Geometry: final body of the model. Coordinates: model frame, mm. A direction names the side the tool comes from. Coordinates: 2 decimals unless noted, no trailing zeros. Loops run counter-clockwise (first coordinate to the right, second up) from the corner with the lowest first, then second, coordinate; pieces in that order, holes last. Notation, with made-up numbers: (14.5, -11.5) -> (44.5, -11.5) arc R27 cw to (44.5, 17.5) -> close; hole circle Ø3 at (-15.5, -30.5). An arc over 180 degrees is marked (long way). One line per item, written item: value. Start each with the question number.
Item 1: Section query D-D on z = 3. Return loops of the section in (x, y), then the cut area to 3 significant figures.
Item 2: Section query C-C on y = 14.95. Give the number of separate pieces and of enclosed holes in the cut face, then the cut area to 3 significant figures.
Item 3: Ray query, probe 1 along Y at (x, z) = (3.2, 0.4); probe 2 along Z at (x, y) = (4.25, 9.5); probe 3 along Y at (x, z) = (3.2, 3.6). Return the intervals inside material, ascending. Write a range as from..to.
Item 4: Set-up query: faces 4 (the flat face through (2, 2, 3.35)), 5 (the flat face through (10.7, 14.8, 0.5)), 6 (the cylindrical face through (11.79, 11.76, 0.49)), 7 (the flat face through (13.353, 9, -2)). Return all of +Z, -Z, +X, -X, +Y, -Y with unobstructed straight access to the full face (end or side cutting, diameter ignored); none if empty.
Item 5: Section query A-A on x = 10.2. Return loops of the section in (y, z).
Item 6: Contact query for flat-ended pins moving along their axis: pin 1 Ø0.6 at (y, z) = (15, 1) entering from -X; pin 2 Ø1.6 at (y, z) = (11.5, -1.5) entering from -X; pin 3 Ø1.2 at (x, y) = (2, 2.5) entering from -Z; pin 4 Ø2 at (x, y) = (3.2, 2.95) entering from +Z. Output: stop coordinate, or through.
Item 7: Mould query, pull axis Y, two halves, no side actions, for faces 1 (the cylindrical face through (4.265, 2.396, 3.646)), 2 (the flat face through (14.24, 8.726, 2.806)), 3 (the flat face through (11.4, 17.1, 0.5)). Classes: +Y half, -Y half, draft (parallel to the pull), parting line (faces both ways), or undercut.
from build123d import *

# Parameters (mm, degrees)
BOSS_EXTRUDE1_DEPTH                             = 15.4
CUT_EXTRUDE2_REACH                              = 25.978
SKETCH3_W                                       = 7.5
SKETCH3_H                                       = 11.5
BOSS_EXTRUDE3_REACH                             = 25.978
SKETCH4_W                                       = 0.8
SKETCH4_H                                       = 6.2
SKETCH4_W_2                                     = 2.8
SKETCH4_H_2                                     = 17.7
SKETCH10_W                                      = 4
SKETCH10_H                                      = 1
CUT_EXTRUDE4_DEPTH                              = 16.3
BOSS_EXTRUDE4_DEPTH                             = 0.8
CSK_FOR_M2_FLAT_HEAD_MACHINE_SCREW3_D           = 2.4
CSK_FOR_M2_FLAT_HEAD_MACHINE_SCREW3_CSINK_D     = 4.4
CSK_FOR_M2_FLAT_HEAD_MACHINE_SCREW3_CSINK_ANGLE = 90
MOVE_FACE1_BY                                   = 0.6
SKETCH3_2_W                                     = 7.5
SKETCH3_2_H                                     = 11.5
BOSS_EXTRUDE6_DEPTH                             = 0.8
CHAMFER1_SIZE                                   = 2.5
CHAMFER1_SIZE2                                  = 4
SKETCH12_W                                      = 2.0475
SKETCH12_H                                      = 3.18
BOSS_EXTRUDE5_DEPTH                             = 17.7
SKETCH11_R                                      = 1.75
CUT_EXTRUDE5_DEPTH                              = 25.580050854
BOSS_EXTRUDE7_DEPTH                             = 1
SKETCH16_W                                      = 8.2
SKETCH16_H                                      = 5.5
CUT_EXTRUDE6_DEPTH                              = 0.5
FILLET5_R                                       = 0.5
FILLET6_R                                       = 0.8


with BuildPart() as part:
    # Sketch2 → Boss-Extrude1 (new body)
    with BuildSketch(Plane(origin=(0, 0, 0), x_dir=(0, 0, -1), z_dir=(1, 0, 0))):
        Polygon((0, 0), (-4.95, 0), (-4.95, 17.7), (-4.15, 17.7), (-4.15, 0.8), (-1, 0.8), (-1, 17.7), (0, 17.7), align=None)
    extrude(amount=BOSS_EXTRUDE1_DEPTH)

    # Sketch3 → Cut-Extrude2 (cut, up to next)
    with BuildSketch(Plane.XY.offset(4.95), mode=Mode.PRIVATE) as cut_extrude2_sk1:
        with Locations((3.75, 11.95)):
            Rectangle(SKETCH3_W, SKETCH3_H)
    cut_extrude2_tool1 = extrude(cut_extrude2_sk1.sketch, amount=-CUT_EXTRUDE2_REACH, mode=Mode.PRIVATE) & part.part
    add(cut_extrude2_tool1.solids().sort_by_distance((3.75, 11.95, 4.95))[0], mode=Mode.SUBTRACT)

    # Sketch4 → Boss-Extrude3 (add, up to next)
    with BuildSketch(Plane.XY.offset(4.95), mode=Mode.PRIVATE) as boss_extrude3_sk1:
        with Locations((0.4, 3.1)):
            Rectangle(SKETCH4_W, SKETCH4_H)
    boss_extrude3_tool1 = extrude(boss_extrude3_sk1.sketch, amount=-BOSS_EXTRUDE3_REACH, mode=Mode.PRIVATE) - part.part
    # Sketch4 → Boss-Extrude3 (add, up to next)
    with BuildSketch(Plane.XY.offset(4.95), mode=Mode.PRIVATE) as boss_extrude3_sk2:
        with Locations((14, 8.85)):
            Rectangle(SKETCH4_W_2, SKETCH4_H_2)
    boss_extrude3_tool2 = extrude(boss_extrude3_sk2.sketch, amount=-BOSS_EXTRUDE3_REACH, mode=Mode.PRIVATE) - part.part
    add(boss_extrude3_tool1.solids().sort_by_distance((0.4, 3.1, 4.95))[0])
    add(boss_extrude3_tool2.solids().sort_by_distance((14, 8.85, 4.95))[0])

    # Sketch10 → Cut-Extrude4 (cut)
    with BuildSketch(Plane(origin=(0, 17.7, 0), x_dir=(1, 0, 0), z_dir=(0, 1, 0))):
        with Locations((10.2, -0.5)):
            Rectangle(SKETCH10_W, SKETCH10_H)
    extrude(amount=-CUT_EXTRUDE4_DEPTH, mode=Mode.SUBTRACT)

    # Sketch6 → Boss-Extrude4 (add)
    with BuildSketch(Plane(origin=(0, 0, 4.15), x_dir=(-1, 0, 0), z_dir=(0, 0, -1))):
        with BuildLine():
            Line((-0.8, 0.8), (-5.05, 0.8))
            Line((-5.05, 0.8), (-5.05, 2.95))
            ThreePointArc((-5.05, 2.95), (-4.508147545, 4.258147545), (-3.2, 4.8))
            Line((-3.2, 4.8), (-0.8, 4.8))
            Line((-0.8, 4.8), (-0.8, 0.8))
        make_face()
    extrude(amount=BOSS_EXTRUDE4_DEPTH)

    # CSK for M2 Flat Head Machine Screw3 (through all)
    with Locations(Plane(origin=(10.2, 14.95, 4.95), x_dir=(0, 1, 0), z_dir=(0, 0, 1))):
        with Locations((0, 0), (-12, 7)):
            CounterSinkHole(CSK_FOR_M2_FLAT_HEAD_MACHINE_SCREW3_D / 2, CSK_FOR_M2_FLAT_HEAD_MACHINE_SCREW3_CSINK_D / 2, counter_sink_angle=CSK_FOR_M2_FLAT_HEAD_MACHINE_SCREW3_CSINK_ANGLE)

    # Move Face1: a face moved inward by 0.6
    extrude(part.faces().sort_by_distance((4.1, 17.7, 0.5))[0], amount=MOVE_FACE1_BY, dir=(0, -1, 0), mode=Mode.SUBTRACT)

    # Sketch3<2> → Boss-Extrude6 (add)
    with BuildSketch(Plane.XY.offset(4.95)):
        with Locations((3.75, 11.95)):
            Rectangle(SKETCH3_2_W, SKETCH3_2_H)
    extrude(amount=-BOSS_EXTRUDE6_DEPTH)

    # Chamfer1
    chamfer1_edges = [part.edges().sort_by_distance(p)[0] for p in [
        (15.4, 8.85, 4.95),
    ]]
    chamfer1_side = [part.faces().sort_by_distance(p)[0] for p in [
        (7.825575812, 8.837442419, 4.95),
    ]]
    chamfer(chamfer1_edges, length=CHAMFER1_SIZE, length2=CHAMFER1_SIZE2, reference=chamfer1_side[0])

    # Sketch12 → Boss-Extrude5 (add)
    with BuildSketch(Plane(origin=(0, 17.7, 0), x_dir=(1, 0, 0), z_dir=(0, 1, 0))):
        with Locations((14.37625, 1.59)):
            Rectangle(SKETCH12_W, SKETCH12_H)
    extrude(amount=-BOSS_EXTRUDE5_DEPTH)

    # Sketch11 → Cut-Extrude5 (cut, through all)
    with BuildSketch(Plane(origin=(0, 0, 4.15), x_dir=(-1, 0, 0), z_dir=(0, 0, -1))):
        with Locations(Location((-10.2, 14.95, 0), (0, 0, 90))):
            Circle(SKETCH11_R)
    extrude(amount=-CUT_EXTRUDE5_DEPTH, mode=Mode.SUBTRACT)

    # Sketch14 → Boss-Extrude7 (add)
    with BuildSketch(Plane(origin=(0, 0, 0), x_dir=(-1, 0, 0), z_dir=(0, 0, -1))):
        with BuildLine():
            Line((-12.2, 17.1), (-12.2, 10.55))
            ThreePointArc((-12.2, 10.55), (-11.78113883, 11.774744871), (-10.7, 12.486491673))
            Line((-10.7, 12.486491673), (-10.7, 17.1))
            Line((-10.7, 17.1), (-12.2, 17.1))
        make_face()
        with BuildLine():
            ThreePointArc((-9.7, 12.486491673), (-8.61886117, 11.774744871), (-8.2, 10.55))
            Line((-8.2, 10.55), (-8.2, 17.1))
            Line((-8.2, 17.1), (-9.7, 17.1))
            Line((-9.7, 17.1), (-9.7, 12.486491673))
        make_face()
    extrude(amount=-BOSS_EXTRUDE7_DEPTH)

    # Sketch16 → Cut-Extrude6 (cut)
    with BuildSketch(Plane.XY.offset(1)):
        with Locations((4.1, 14.35)):
            Rectangle(SKETCH16_W, SKETCH16_H)
    extrude(amount=-CUT_EXTRUDE6_DEPTH, mode=Mode.SUBTRACT)

    # Fillet5
    fillet5_edges = [part.edges().sort_by_distance(p)[0] for p in [
        (12.9, 8.85, 4.95),
    ]]
    fillet(fillet5_edges, radius=FILLET5_R)

    # Fillet6
    fillet6_edges = [part.edges().sort_by_distance(p)[0] for p in [
        (0.8, 5.5, 4.15),
        (0, 17.1, 0.25),
        (0, 17.7, 4.55),
        (0.4, 6.2, 4.15),
        (8.2, 11.6, 0.75),
        (0.4, 6.2, 1),
        (12.6, 9.25, 4.15),
    ]]
    fillet(fillet6_edges, radius=FILLET6_R)


solid = part.part
Reply:
1. outline: (0, 0) -> (14.12, 0) -> (14.12, 17.7) -> (12.6, 17.7) -> (12.6, 0.8) -> (0.8, 0.8) -> (0.8, 6.2) -> (0, 6.2) -> close
1. area: 41.3 mm²
2. separate pieces: 3
2. enclosed holes: 0
2. area: 30.1 mm²
3. probe 1: y = 0..1.75, 4.15..17.1
3. probe 2: z = 0..1, 4.15..4.95
3. probe 3: y = 0..1.75, 4.15..4.8
4. face 4: +Y
4. face 5: -Z, +Y
4. face 6: -Z
4. face 7: -Z, -X, +Y, -Y
5. outline: (0, 0) -> (1.4, 0) -> (1.4, 1) -> (0.8, 1) -> (0.8, 4.15) -> (13.2, 4.15) -> (13.2, 4.5) -> (12.75, 4.95) -> (0, 4.95) -> close; (16.7, 4.15) -> (17.7, 4.15) -> (17.7, 4.95) -> (17.15, 4.95) -> (16.7, 4.5) -> close
6. pin 1: stops at x = 8.2
6. pin 2: stops at x = 13.35
6. pin 3: stops at z = 0
6. pin 4: passes through
7. face 1: undercut
7. face 2: draft
7. face 3: +Y half
